Part print with two shaded views. Sizes in mm from the minimum x, y, z corner. Give positions to 0.01 mm unless a question says otherwise; leave off trailing zeros. Write each loop counter-clockwise with the first axis right and the second up, starting at its lowest first coordinate (ties: lowest second). Pieces come first, ordered by that corner, then holes.
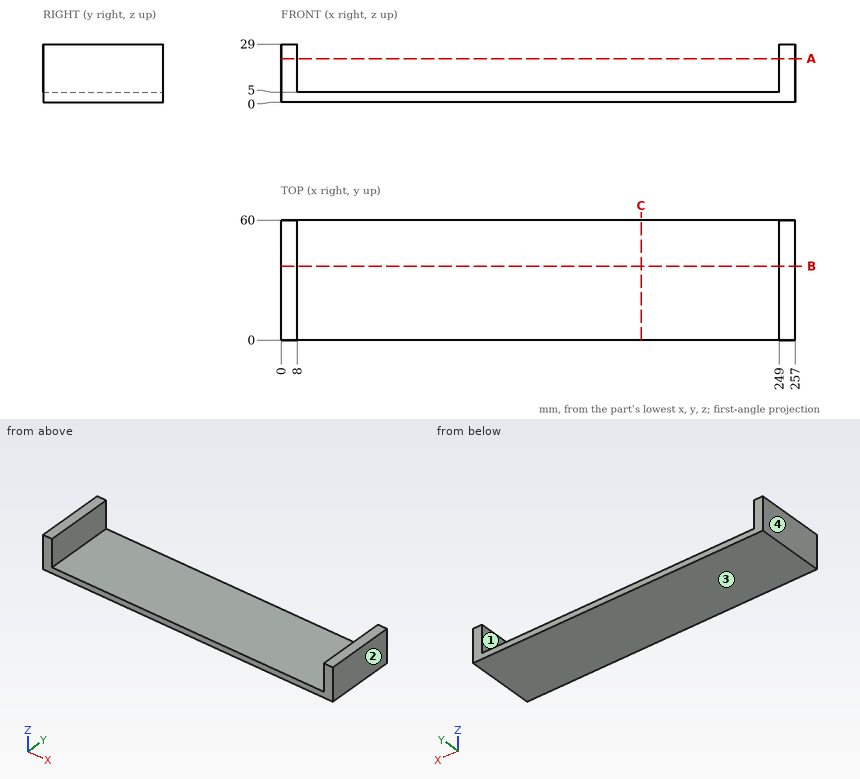
1) Pin check, flat tip, straight feed: pin 1 Ø8 at (x, y) = (90, 36) entering from +Z. Stop position of the tip, or through.
Answers follow:
pin 1: stops at z = 5
2) Saw through at A-A, the plane z = 21.75. Write the cut outline in (x, y).
Answers follow:
outline: (0, 0) - (8, 0) - (8, 60) - (0, 60) - close; (249, 0) - (257, 0) - (257, 60) - (249, 60) - close
3) Wall check: L1, parallel to X at y = 22, z = 6.25; L2, parallel to Z at x = 237, y = 12.5. Give the ranges that are in metal, low to high.
Answers follow:
L1: x = 0 to 8, 249 to 257
L2: z = 0 to 5
4) Saw through at B-B, the plane y = 37. Write the cut outline in (x, z).
Answers follow:
outline: (0, 0) - (257, 0) - (257, 29) - (249, 29) - (249, 5) - (8, 5) - (8, 29) - (0, 29) - close
5) Two-plate mould, pull along X, no slides. Class the marked faces 1, 2, 3 and 4: +X half, -X half, draft (parallel to the pull), parting line (faces both ways), or undercut.
Answers follow:
face 1: undercut
face 2: +X half
face 3: draft
face 4: -X half
6) Saw through at C-C, the plane x = 180. Write the cut outline in (y, z).
Answers follow:
outline: (0, 0) - (60, 0) - (60, 5) - (0, 5) - close
